```python
from build123d import *

# Parameters (mm, degrees)
F0_R     = 11
F1_DEPTH = 66.3
F3_DEPTH = 2
F4_R     = 2
F5_DEPTH = 16.2
F6_W     = 2.6457513111
F6_H     = 0.5
F7_DEPTH = 12
F9_D     = 1.5
F9_DEPTH = 10
F9_TIP   = 0.4506454643


with BuildPart() as f1:
    # F0 (on Top) → F1 (new body)
    with BuildSketch(Plane.XY):
        Circle(F0_R)
    extrude(amount=-F1_DEPTH)

    # F2 (on face) → F3 (join)
    with BuildSketch(Plane.XY):
        with BuildLine():
            ThreePointArc((6, 3.6055512755), (0, 7), (-6, 3.6055512755))
            Line((-6, 3.6055512755), (-6, -3.6055512755))
            ThreePointArc((-6, -3.6055512755), (0, -7), (6, -3.6055512755))
            Line((6, -3.6055512755), (6, 3.6055512755))
        make_face()
    extrude(amount=F3_DEPTH)

    # F4 (on face) → F5 (join)
    with BuildSketch(Plane.XY.offset(2)):
        Circle(F4_R)
    extrude(amount=F5_DEPTH)

    # F6 (on face) → F7 (cut)
    with BuildSketch(Plane.XY.offset(18.2)):
        with Locations((0, 1.75)):
            Rectangle(F6_W, F6_H)
    extrude(amount=-F7_DEPTH, mode=Mode.SUBTRACT)

    # F9
    with Locations(Plane.XY):
        with Locations((-6.3639610307, 6.3639610307), (-6.3639610307, -6.3639610307), (6.3639610307, 6.3639610307), (6.3639610307, -6.3639610307)):
            Hole(F9_D / 2, depth=F9_DEPTH)
            with Locations((0, 0, -(F9_DEPTH + F9_TIP / 2))):  # 118° drill point
                Cone(0, F9_D / 2, F9_TIP, mode=Mode.SUBTRACT)


solid = f1.part
```
Geometry: final body of the model. Coordinates: model frame, mm. A direction names the side the tool comes from. Round coordinates to 2 decimals unless told otherwise and drop trailing zeros. Write each loop counter-clockwise with the first axis right and the second up, starting at its lowest first coordinate (ties: lowest second). Pieces come first, ordered by that corner, then holes.
Item 1: Section query A-A (y = 0). Return loops of the section in (x, z), plus the area to 3 significant figures.
Item 2: Material intervals for L1, parallel to Z at x = -8.25, y = 7; L2, parallel to Z at x = -2, y = 2.75; L3, parallel to Y at x = -0.5, z = -60.5, sorted ascending.
Item 3: Section query D-D (z = -26.5). Return loops of the section in (x, y), plus the area to 3 significant figures.
Item 4: Set-up query: faces 1 (the face through (0, 7, 1)), 2 (the face through (0, -7, 1)), 3 (the face through (7.113, 6.397, -5.07)), 4 (the face through (-6, 0, 1)). Return all of +Z, -Z, +X, -X, +Y, -Y with unobstructed straight access to the full face (end or side cutting, diameter ignored); none if empty.
Item 5: Mould query, pull axis Y, two halves, no side actions, for faces 5 (the face through (6.23, -6.36, -10.37)), 6 (the face through (7, 0, 0)), 7 (the face through (0, 1.5, 12)). Classes: +Y half, -Y half, draft (parallel to the pull), parting line (faces both ways), or undercut.
Item 6: Section query C-C (z = -8.5). Return loops of the section in (x, y).
Item 7: Pin query (flat end, axial travel): P1, Ø0.9, axis at x = -6.36, y = 6.36, coming from the +Z side; P2, Ø10, axis at x = 6, z = -5.5, coming from the -Y side; P3, Ø3, axis at x = -4.5, y = 4.5, coming from the +Z side. Return the tip coordinate at first contact, or that it passes through.
Item 8: Section query B-B (x = 0). Return loops of the section in (y, z), plus the area to 3 significant figures.
Completed:
1. outline: (-11, -66.3) - (11, -66.3) - (11, 0) - (6, 0) - (6, 2) - (2, 2) - (2, 18.2) - (-2, 18.2) - (-2, 2) - (-6, 2) - (-6, 0) - (-11, 0) - close
1. area: 1,550 mm2
2. L1: z = -66.3 to 0
2. L2: z = -66.3 to 2
2. L3: y = -10.99 to 10.99
3. outline: circle Ø22 at (0, 0)
3. area: 380 mm2
4. face 1: +Z, +Y
4. face 2: +Z, -Y
4. face 3: +Z
4. face 4: +Z, -X, +Y, -Y
5. face 5: undercut
5. face 6: draft
5. face 7: +Y half
6. outline: circle Ø22 at (0, 0); hole circle Ø1.5 at (-6.36, -6.36); hole circle Ø1.5 at (-6.36, 6.36); hole circle Ø1.5 at (6.36, -6.36); hole circle Ø1.5 at (6.36, 6.36)
7. P1: stops at z = -10.18
7. P2: stops at y = -10.95
7. P3: stops at z = 2
8. outline: (-11, -66.3) - (11, -66.3) - (11, 0) - (7, 0) - (7, 2) - (2, 2) - (2, 6.2) - (1.5, 6.2) - (1.5, 18.2) - (-2, 18.2) - (-2, 2) - (-7, 2) - (-7, 0) - (-11, 0) - close
8. area: 1,550 mm2
